```python
from build123d import *

# Parameters (mm, degrees)
SKETCH1_R           = 3.05
SKETCH1_R_2         = 2.5
BOSS_EXTRUDE1_DEPTH = 4
SKETCH2_R           = 1.3
CUT_EXTRUDE1_DEPTH  = 4
BOSS_EXTRUDE2_DEPTH = 4
BOSS_EXTRUDE3_DEPTH = 4
FILLET1_R           = 1
FILLET9_R           = 0.5
FILLET10_R          = 2


with BuildPart() as part:
    # Sketch1 → Boss-Extrude1 (new body)
    with BuildSketch(Plane(origin=(0, 0, 0), x_dir=(1, 0, 0), z_dir=(0, 1, 0))):
        with BuildLine():
            Line((-4.531642246, 17.7995776), (-7.838367177, 1.6))
            ThreePointArc((-7.838367177, 1.6), (0, -8), (7.838367177, 1.6))
            Line((7.838367177, 1.6), (4.531642246, 17.7995776))
            ThreePointArc((4.531642246, 17.7995776), (0, 21.499648), (-4.531642246, 17.7995776))
        make_face()
        with Locations((0, 16.87456)):
            Circle(SKETCH1_R, mode=Mode.SUBTRACT)
        Circle(SKETCH1_R_2, mode=Mode.SUBTRACT)
    extrude(amount=BOSS_EXTRUDE1_DEPTH)

    # Sketch2 → Cut-Extrude1 (cut)
    with BuildSketch(Plane(origin=(0, 4, 0), x_dir=(1, 0, 0), z_dir=(0, 1, 0))):
        with Locations((0, 6.35)):
            Circle(SKETCH2_R)
        with Locations((6.35, 0)):
            Circle(SKETCH2_R)
        with Locations((0, -6.35)):
            Circle(SKETCH2_R)
        with Locations((-6.35, 0)):
            Circle(SKETCH2_R)
    extrude(amount=-CUT_EXTRUDE1_DEPTH, mode=Mode.SUBTRACT)

    # Sketch3 → Boss-Extrude2 (add)
    with BuildSketch(Plane(origin=(0, 4, 0), x_dir=(1, 0, 0), z_dir=(0, 1, 0))):
        with BuildLine():
            Line((-7.838367177, 1.6), (-6.8136721, 6.619960159))
            ThreePointArc((-6.8136721, 6.619960159), (0, -9.5), (6.8136721, 6.619960159))
            Line((6.8136721, 6.619960159), (7.838367177, 1.6))
            ThreePointArc((7.838367177, 1.6), (0, -8), (-7.838367177, 1.6))
        make_face()
    extrude(amount=-BOSS_EXTRUDE2_DEPTH)

    # Sketch4 → Boss-Extrude3 (add)
    with BuildSketch(Plane(origin=(0, 4, 0), x_dir=(1, 0, 0), z_dir=(0, 1, 0))):
        with BuildLine():
            Line((10.392304845, 8.510381451), (6.42779147, 8.510381451))
            Line((6.42779147, 8.510381451), (6.8136721, 6.619960159))
            Line((6.8136721, 6.619960159), (1.793071605, 1.742094779))
            ThreePointArc((1.793071605, 1.742094779), (1.994303817, 1.507565019), (2.165063509, 1.25))
            Line((2.165063509, 1.25), (5.073143183, 2.928980582))
            Line((5.073143183, 2.928980582), (8.943807158, 3.20286021))
            Line((8.943807158, 3.20286021), (10.361060865, 5.990375719))
            Line((10.361060865, 5.990375719), (11.642304845, 8.510381451))
            Line((11.642304845, 8.510381451), (10.392304845, 8.510381451))
        make_face()
    extrude(amount=-BOSS_EXTRUDE3_DEPTH)

    # Fillet1
    fillet1_edges = [part.edges().sort_by_distance(p)[0] for p in [
        (-6.8136721, 2, -6.619960159),
    ]]
    fillet(fillet1_edges, radius=FILLET1_R)

    # Fillet9
    fillet9_edges = [part.edges().sort_by_distance(p)[0] for p in [
        (11.642304845, 2, -8.510381451),
    ]]
    fillet(fillet9_edges, radius=FILLET9_R)

    # Fillet10
    fillet10_edges = [part.edges().sort_by_distance(p)[0] for p in [
        (6.42779147, 2, -8.510381451),
    ]]
    fillet(fillet10_edges, radius=FILLET10_R)


solid = part.part
```
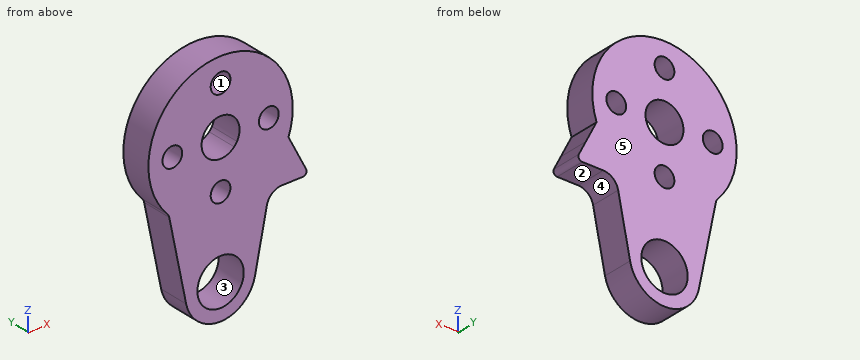
Input: part model. Units: mm. Frame: model coordinates. Face numbers are marked on the shaded views. A direction names the side the tool comes from. Round coordinates to 2 decimals unless told otherwise and drop trailing zeros. Loops run counter-clockwise (first coordinate to the right, second up) from the corner with the lowest first, then second, coordinate; pieces in that order, holes last.
1) Section query D-D on x = 7.25. Return the cut outline in (y, z).
Ans:
outline: (0, -8.68) - (4, -8.68) - (4, -0.94) - (0, -0.94) - close; (0, 0.94) - (4, 0.94) - (4, 6.14) - (0, 6.14) - close
2) Section query B-B on x = 0. Return the cut outline in (y, z).
Ans:
outline: (0, -21.5) - (4, -21.5) - (4, -19.92) - (0, -19.92) - close; (0, -13.82) - (4, -13.82) - (4, -7.65) - (0, -7.65) - close; (0, -5.05) - (4, -5.05) - (4, -2.5) - (0, -2.5) - close; (0, 2.5) - (4, 2.5) - (4, 5.05) - (0, 5.05) - close; (0, 7.65) - (4, 7.65) - (4, 9.5) - (0, 9.5) - close
3) Section query A-A on z = 0. Return the cut outline in (x, y), plus the area to 3 significant figures.
Ans:
outline: (-9.5, 0) - (-7.65, 0) - (-7.65, 4) - (-9.5, 4) - close; (-5.05, 0) - (-2.5, 0) - (-2.5, 4) - (-5.05, 4) - close; (2.5, 0) - (5.05, 0) - (5.05, 4) - (2.5, 4) - close; (7.65, 0) - (9.5, 0) - (9.5, 4) - (7.65, 4) - close
area: 35.2 mm2
4) Set-up query: the marked faces 1 and 2. Return all of +Z, -Z, +X, -X, +Y, -Y with unobstructed straight access to the full face (end or side cutting, diameter ignored); none if empty.
Ans:
face 1: +Y, -Y
face 2: -Z, +X, +Y, -Y
5) Pin query (flat end, axial travel): pin 1 (1.5 mm diameter, centred on y = 1.5, z = -4, fed in from -X); pin 2 (3 mm diameter, centred on x = 0, z = 0, fed in from -Y). Return the tip coordinate at first contact, or that it passes through.
Ans:
pin 1: stops at x = -8.93
pin 2: passes through
6) Pull-direction query (X, two-part tool) for the marked faces 3, 4 and 5; classes: released by +X, released by -X, zero draft, split by the parting line, or undercut.
Ans:
face 3: undercut
face 4: released by +X
face 5: zero draft
7) Material intervals for line 1 (X direction, y = 2.85, z = 0); line 2 (Z direction, x = 0, y = 2.3); line 3 (Z direction, x = 2, y = 2), sorted ascending.
Ans:
line 1: x = -9.5 to -7.65, -5.05 to -2.5, 2.5 to 5.05, 7.65 to 9.5
line 2: z = -21.5 to -19.92, -13.82 to -7.65, -5.05 to -2.5, 2.5 to 5.05, 7.65 to 9.5
line 3: z = -21.04 to -19.18, -14.57 to -1.5, 1.5 to 9.29
8) Section query C-C on z = -16.5. Return the cut outline in (x, y).
Ans:
outline: (-4.8, 0) - (-3.03, 0) - (-3.03, 4) - (-4.8, 4) - close; (3.03, 0) - (4.8, 0) - (4.8, 4) - (3.03, 4) - close
